Check sheet for the drawn part. Datum: minimum x, y, z corner. Units: mm. A direction names the side the tool comes from. Coordinates: 2 decimals unless noted, no trailing zeros. Order: outer loops, then holes, each group sorted by start corner. A loop starts at its lowest first (then second) coordinate and runs counter-clockwise, first axis right, second up. Notation, with made-up numbers: M -32,87 L -6,87 A35 ccw -6,122 Z; hole C -2,-29.75 d11. An arc over 180 degrees is marked long. Return JSON: item names as keys, results as strings. Group by question number.
Q1. Thickness scan on probe 1 along X at (y, z) = (1, 1.5); probe 2 along Z at (x, y) = (18, 0.9); probe 3 along Y at (x, z) = (10, 1.6). Record the ranges inside material, lowest first.
Q2. Mould release check, pull along X, two halves, no side actions. Record for the marked faces 4, 5 and 6: pulls with the +X half, pulls with the -X half, needs draft (parallel to the pull), parting line crosses it, or undercut.
Q3. Go/stop test with flat-tipped pins: pin 1 Ø0.9 at (x, z) = (1.5, 2) entering from +Y; pin 2 Ø1 at (y, z) = (13, 0.5) entering from +X. Record where each tip stops, or that it passes through.
Q4. Section check D-D, the plane x = 4.25. Enter the section's corners in (y, z).
Q5. Section check C-C, the plane y = 9.5. Enter the section's corners in (x, z).
Q6. Section check B-B, the plane x = 18. Enter the section's corners in (y, z), then the cut area to 3 significant figures.
Q7. Access from +Z, -Z, +X, -X, +Y, -Y to the whole of each face (thin tool, end or side, straight path). Record for the marked faces 1, 2 and 3.
Q8. Section check A-A, the plane z = 1.5. Enter the section's corners in (x, y).
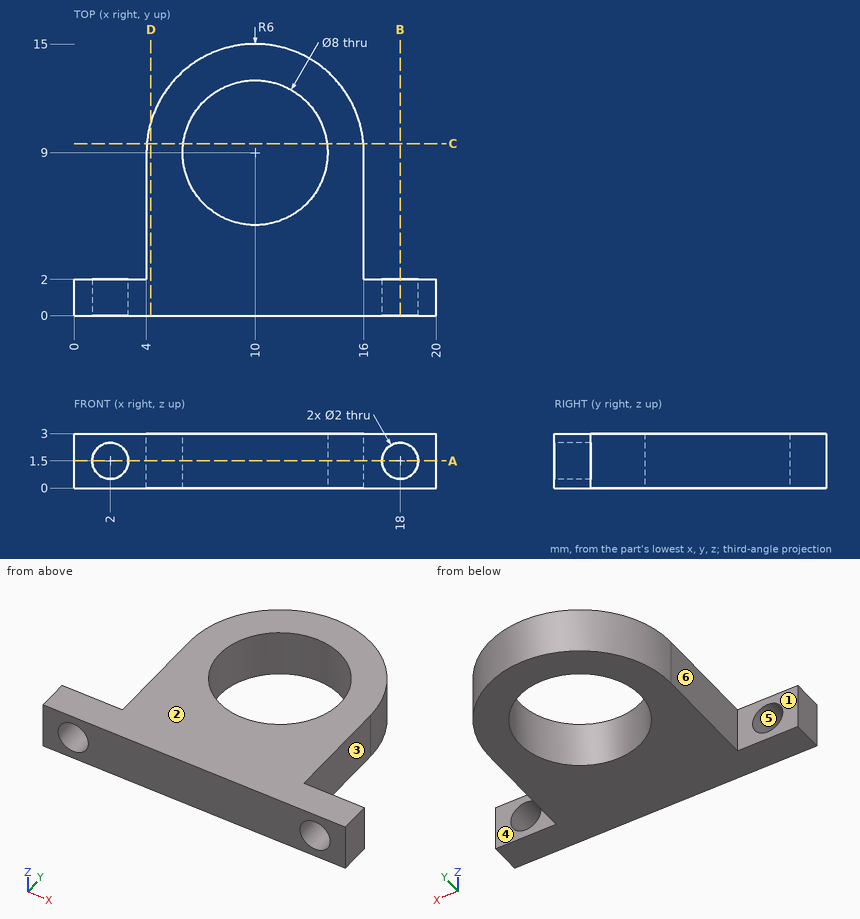
Numbers:
{
 "1": {"probe 1": "x = 0 to 1, 3 to 17, 19 to 20", "probe 2": "z = 0 to 0.5, 2.5 to 3", "probe 3": "y = 0 to 5, 13 to 15"},
 "2": {"face 4": "needs draft", "face 5": "undercut", "face 6": "pulls with the -X half"},
 "3": {"pin 1": "stops at y = 2", "pin 2": "stops at x = 14.87"},
 "4": {"outline": "M 0,0 L 10.71,0 L 10.71,3 L 0,3 Z"},
 "5": {"outline": "M 4.02,0 L 6.03,0 L 6.03,3 L 4.02,3 Z; M 13.97,0 L 15.98,0 L 15.98,3 L 13.97,3 Z"},
 "6": {"outline": "M 0,0 L 2,0 L 2,0.5 L 0,0.5 Z; M 0,2.5 L 2,2.5 L 2,3 L 0,3 Z", "area": "2.00 mm2"},
 "7": {"face 1": "+Z, -Z, -X, +Y", "face 2": "+Z, +X, -X, +Y, -Y", "face 3": "+Z, -Z, +X, +Y"},
 "8": {"outline": "M 0,0 L 1,0 L 1,2 L 0,2 Z; M 3,0 L 17,0 L 17,2 L 16,2 L 16,9 A6 ccw 4,9 L 4,2 L 3,2 Z; M 19,0 L 20,0 L 20,2 L 19,2 Z; hole C 10,9 d8"}
}
